Model file for the job. Use its own axes, mm. A direction names the side the tool comes from. Coordinates: 2 decimals unless noted, no trailing zeros. Order: outer loops, then holes, each group sorted by start corner. A loop starts at its lowest first (then second) coordinate and runs counter-clockwise, first axis right, second up. Notation, with made-up numbers: (-5.75, 26) -> (41.25, 26) arc R22 cw to (41.25, 53) -> close; hole circle Ø11 at (-15, -21.75). An arc over 180 degrees is marked (long way). Write item = value, one per line. Start each with the question number.
Q1. Cut at A-A, the plane z = 15. List the corners of the cut face in (x, y), plus the area to 3 significant figures.
Q2. Mould opens along X. For faces 1 (the face through (14.37, -37.18, 16.39)), 2 (the face through (-1, 1, 0)), 3 (the face through (-80.608, 3.548, 12.611)) say: +X half, -X half, draft (parallel to the pull), parting line (faces both ways), or undercut.
Q3. Wall check: line 1 (Y direction, x = -11, z = 17.75); line 2 (X direction, y = -6, z = 17.25); line 3 (X direction, y = -26, z = 8). Give the ranges that are in metal, low to high. Write a range as from..to.
Q4. 3-axis set-ups, long thin cutter, end or side, ignore diameter. For faces 4 (the face through (-15.4, 29.4, 25.4)), 5 (the face through (-16.095, 38.216, 16.386)): which of +Z, -Z, +X, -X, +Y, -Y reach the whole face in a straight line?
Q5. Cut at B-B, the plane x = 0. List the corners of the cut face in (y, z).
Q6. Flat gauge pins, fed straight in: pin 1 (6 mm diameter, centred on x = -62, y = -46.5, fed in from -Z); pin 2 (10 mm diameter, centred on y = 33, z = 11.5, fed in from +X); pin 3 (1.5 mm diameter, centred on y = 46, z = 6, fed in from +X). Where does each tip first touch, or does it go through?
from build123d import *

# Parameters (mm, degrees)
F0_R     = 80.6856028543
F1_DEPTH = 25.4
F2_DEPTH = 7.62


# Not quite as in the source:
# - a fillet or chamfer that OpenCascade refuses, or shapes differently, is made with other operations: its cross-section is extruded or revolved along the edge and cut away or added


with BuildPart() as f1:
    # F0 (on Top) → F1 (new body)
    with BuildSketch(Plane.XY):
        Circle(F0_R)
        with BuildLine():
            ThreePointArc((65.4481636504, 35.6006994652), (72.2046857665, 18.3672338959), (74.5041738939, 0))
            ThreePointArc((74.5041738939, 0), (-18.3672338959, -72.2046857665), (-65.4481636504, 35.6006994652))
            ThreePointArc((-65.4481636504, 35.6006994652), (0, 74.5041738939), (65.4481636504, 35.6006994652))
        make_face(mode=Mode.SUBTRACT)
        with BuildLine():
            Line((60.4875776026, 27.0912961706), (65.4481636504, 35.6006994652))
            ThreePointArc((65.4481636504, 35.6006994652), (0, 74.5041738939), (-65.4481636504, 35.6006994652))
            Line((-65.4481636504, 35.6006994652), (-60.4875776026, 27.0912961706))
            ThreePointArc((-60.4875776026, 27.0912961706), (-53.0522524477, -16.0833720047), (-18.6689998955, -43.2334728539))
            Line((-18.6689998955, -43.2334728539), (-10.1934868934, -31.2953587769))
            ThreePointArc((-10.1934868934, -31.2953587769), (-32.8922648635, -1.1855666041), (-12.4201237339, 30.4802753015))
            Line((-12.4201237339, 30.4802753015), (-19.8746794874, 46.1712545885))
            ThreePointArc((-19.8746794874, 46.1712545885), (-0.0120295356, 50.8915609087), (19.8259803172, 46.0687484571))
            Line((19.8259803172, 46.0687484571), (12.4201237339, 30.4802753015))
            ThreePointArc((12.4201237339, 30.4802753015), (27.3138970192, 18.3645769254), (32.9136241703, 0))
            ThreePointArc((32.9136241703, 0), (26.6346696302, -19.3365206207), (10.1934868934, -31.2953587769))
            Line((10.1934868934, -31.2953587769), (18.6689998955, -43.2334728539))
            ThreePointArc((18.6689998955, -43.2334728539), (53.0522524477, -16.0833720047), (60.4875776026, 27.0912961706))
        make_face()
    extrude(amount=F1_DEPTH)

    # F0 (on Top) → F2 (join)
    with BuildSketch(Plane.XY):
        with BuildLine():
            ThreePointArc((-10.1934868934, -31.2953587769), (0, -32.9136241703), (10.1934868934, -31.2953587769))
            ThreePointArc((10.1934868934, -31.2953587769), (26.6346696302, -19.3365206207), (32.9136241703, 0))
            ThreePointArc((32.9136241703, 0), (27.3138970192, 18.3645769254), (12.4201237339, 30.4802753015))
            ThreePointArc((12.4201237339, 30.4802753015), (0, 32.9136241703), (-12.4201237339, 30.4802753015))
            ThreePointArc((-12.4201237339, 30.4802753015), (-32.8922648635, -1.1855666041), (-10.1934868934, -31.2953587769))
        make_face()
        with BuildLine():
            Line((-19.8746794874, 46.1712545885), (-12.4201237339, 30.4802753015))
            ThreePointArc((-12.4201237339, 30.4802753015), (0, 32.9136241703), (12.4201237339, 30.4802753015))
            Line((12.4201237339, 30.4802753015), (19.8259803172, 46.0687484571))
            ThreePointArc((19.8259803172, 46.0687484571), (-0.0120295356, 50.8915609087), (-19.8746794874, 46.1712545885))
        make_face()
        with BuildLine():
            ThreePointArc((-65.4481636504, 35.6006994652), (-18.3672338959, -72.2046857665), (74.5041738939, 0))
            ThreePointArc((74.5041738939, 0), (72.2046857665, 18.3672338959), (65.4481636504, 35.6006994652))
            Line((65.4481636504, 35.6006994652), (60.4875776026, 27.0912961706))
            ThreePointArc((60.4875776026, 27.0912961706), (53.0522524477, -16.0833720047), (18.6689998955, -43.2334728539))
            Line((18.6689998955, -43.2334728539), (10.1934868934, -31.2953587769))
            ThreePointArc((10.1934868934, -31.2953587769), (0, -32.9136241703), (-10.1934868934, -31.2953587769))
            Line((-10.1934868934, -31.2953587769), (-18.6689998955, -43.2334728539))
            ThreePointArc((-18.6689998955, -43.2334728539), (-53.0522524477, -16.0833720047), (-60.4875776026, 27.0912961706))
            Line((-60.4875776026, 27.0912961706), (-65.4481636504, 35.6006994652))
        make_face()
    extrude(amount=F2_DEPTH)

    # F3: fillet of radius 6.35 on 2 edges, made by hand

    # F3_s1 → F3_t2 (revolve, cut)
    with BuildSketch(Plane.XZ):
        with BuildLine():
            ThreePointArc((80.6856028543, 19.05), (78.8257309148, 23.5401280605), (74.3356028543, 25.4))
            Line((74.3356028543, 25.4), (74.3356028543, 25.527))
            Line((74.3356028543, 25.527), (80.8126028543, 25.527))
            Line((80.8126028543, 25.527), (80.8126028543, 19.05))
            Line((80.8126028543, 19.05), (80.6856028543, 19.05))
        make_face()
    revolve(axis=Axis((0, 0, 25.4), (0, 0, 1)), mode=Mode.SUBTRACT)

    # F3_s3 → F3_t4 (revolve, cut)
    with BuildSketch(Plane.XZ):
        with BuildLine():
            ThreePointArc((80.6856028543, 6.35), (78.8257309148, 1.8598719395), (74.3356028543, 0))
            Line((74.3356028543, 0), (74.3356028543, -0.127))
            Line((74.3356028543, -0.127), (80.8126028543, -0.127))
            Line((80.8126028543, -0.127), (80.8126028543, 6.35))
            Line((80.8126028543, 6.35), (80.6856028543, 6.35))
        make_face()
    revolve(axis=Axis((0, 0, 0), (0, 0, 1)), mode=Mode.SUBTRACT)


solid = f1.part
Here are the results:
q1.outline = circle Ø161.37 at (0, 0); hole (-65.45, 35.6) arc R74.5 ccw (long way) to (65.45, 35.6) -> (60.49, 27.09) arc R61.22 cw to (18.67, -43.23) -> (10.19, -31.3) arc R32.91 ccw to (12.42, 30.48) -> (19.83, 46.07) arc R43.68 ccw to (-19.87, 46.17) -> (-12.42, 30.48) arc R32.91 ccw to (-10.19, -31.3) -> (-18.67, -43.23) arc R61.22 cw to (-60.49, 27.09) -> close
q1.area = 10,700 mm²
q2.face_1 = undercut
q2.face_2 = draft
q2.face_3 = parting line
q3.line_1 = -79.93..-73.69, -32.43..-31.02, 49.52..79.93
q3.line_2 = -80.46..-74.26, -57.86..-32.36, 32.36..57.86, 74.26..80.46
q3.line_3 = -76.38..-69.82, -45.71..-20.18, 20.18..45.71, 69.82..76.38
q4.face_4 = +Z, +X, -X, +Y, -Y
q4.face_5 = +Z
q5.outline = (-80.69, 6.35) arc R6.35 ccw to (-74.34, 0) -> (74.34, 0) arc R6.35 ccw to (80.69, 6.35) -> (80.69, 19.05) arc R6.35 ccw to (74.34, 25.4) -> (50.89, 25.4) -> (50.89, 7.62) -> (-74.5, 7.62) -> (-74.5, 25.4) arc R6.35 ccw to (-80.69, 19.05) -> close
q6.pin_1 = 0
q6.pin_2 = 75.67
q6.pin_3 = 66.79
